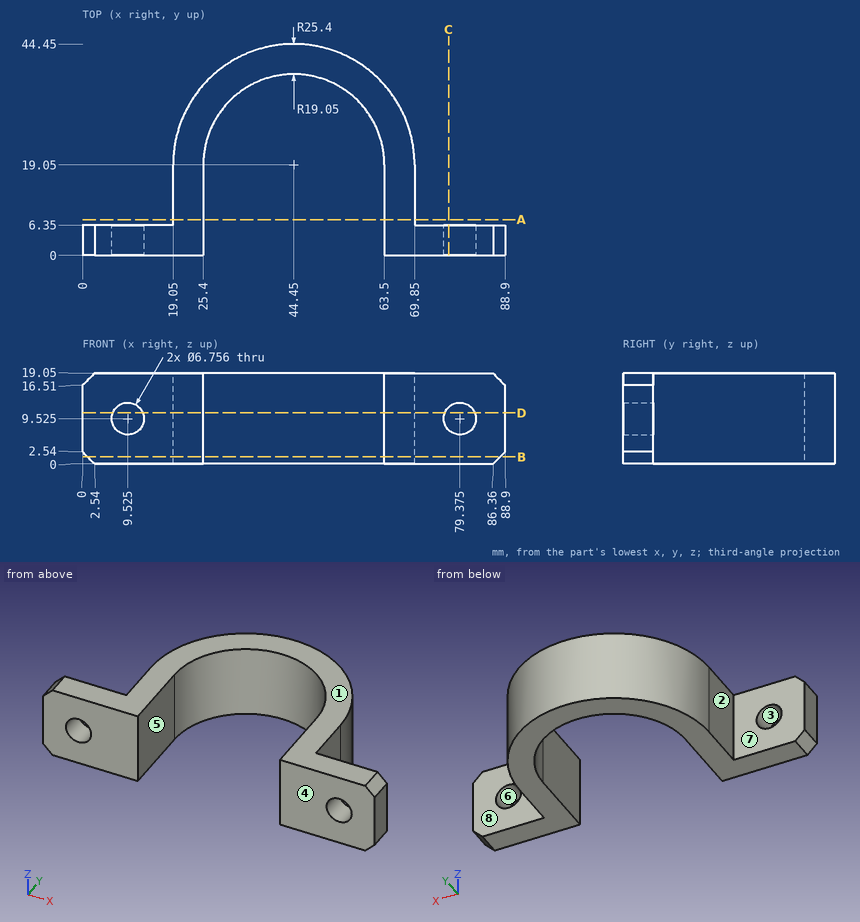
Study the drawing (mm; zero at the part's minimum x, y, z) and answer. A direction names the side the tool comes from. Round coordinates to 2 decimals unless told otherwise and drop trailing zeros. Loops run counter-clockwise (first coordinate to the right, second up) from the corner with the lowest first, then second, coordinate; pieces in that order, holes last.
Q1. Section B-B, the plane z = 1.5 is taken. Determine the outline of the cut face in (x, y), then the cut area to 3 significant figures.
Q2. Section D-D, the plane z = 10.75 is taken. Determine the outline of the cut face in (x, y).
Q3. Section C-C, the plane x = 77 is taken. Determine the outline of the cut face in (y, z).
Q4. Which of the six approach directions +Z, -Z, +X, -X, +Y, -Y give full straight-line access (tool end or side, diameter ignored) to the marked faces 4, 5, 6, 7 and 8?
Q5. Given pin 1 Ø3 at (y, z) = (18, 12.5) entering from +X; pin 2 Ø5.5 at (x, z) = (79.375, 9.525) entering from -Y; pin 3 Ø4 at (x, z) = (57.5, 3.5) entering from +Y; pin 4 Ø5.5 at (x, z) = (5.5, 6.5) entering from +Y, each flat-ended and moving along its own axis, determine where each tip first touches the part or whether it passes through.
Q6. Find the intervals of material crossed by line 1 (X direction, y = 8, z = 12.5); line 2 (X direction, y = 30.5, z = 3) (1 decimal); line 3 (Y direction, x = 4, z = 10), in increasing order.
Q7. Section A-A, the plane y = 7.5 is taken. Determine the outline of the cut face in (x, z).
Q8. For a pull along Z with two mould halves and no side action, classify the marked faces 1, 2 and 3 as released by +Z, released by -Z, zero draft, split by the parting line, or undercut.
Completed:
1. outline: (1.04, 0) - (25.4, 0) - (25.4, 19.05) arc R19.05 cw to (63.5, 19.05) - (63.5, 0) - (87.86, 0) - (87.86, 6.35) - (69.85, 6.35) - (69.85, 19.05) arc R25.4 ccw to (19.05, 19.05) - (19.05, 6.35) - (1.04, 6.35) - close
1. area: 914 mm2
2. outline: (0, 0) - (6.38, 0) - (6.38, 6.35) - (0, 6.35) - close; (12.67, 0) - (25.4, 0) - (25.4, 19.05) arc R19.05 cw to (63.5, 19.05) - (63.5, 0) - (76.23, 0) - (76.23, 6.35) - (69.85, 6.35) - (69.85, 19.05) arc R25.4 ccw to (19.05, 19.05) - (19.05, 6.35) - (12.67, 6.35) - close; (82.52, 0) - (88.9, 0) - (88.9, 6.35) - (82.52, 6.35) - close
3. outline: (0, 0) - (6.35, 0) - (6.35, 7.12) - (0, 7.12) - close; (0, 11.93) - (6.35, 11.93) - (6.35, 19.05) - (0, 19.05) - close
4. face 4: +Z, -Z, +X, -X, -Y
4. face 5: +Z, -Z, -Y
4. face 6: +Y, -Y
4. face 7: +Z, -Z, -X, +Y
4. face 8: +Z, -Z, +X, +Y
5. pin 1: stops at x = 69.85
5. pin 2: passes through
5. pin 3: stops at y = 41.92
5. pin 4: stops at y = 6.35
6. line 1: x = 19.05 to 25.4, 63.5 to 69.85
6. line 2: x = 21.8 to 29.2, 59.7 to 67.1
6. line 3: y = 0 to 6.35
7. outline: (19.05, 0) - (25.4, 0) - (25.4, 19.05) - (19.05, 19.05) - close; (63.5, 0) - (69.85, 0) - (69.85, 19.05) - (63.5, 19.05) - close
8. face 1: released by +Z
8. face 2: zero draft
8. face 3: undercut
